The figure shows three views and two pictorial views of one solid part (mm, origin at its lowest corner). Answer the questions. Coordinates: 2 decimals unless noted, no trailing zeros. Order: outer loops, then holes, each group sorted by start corner. A loop starts at its lowest first (then second) coordinate and runs counter-clockwise, first axis right, second up. Notation, with made-up numbers: (11, 40) - (58, 40) arc R28 ccw to (58, 64) - close; hole circle Ø2 at (73.5, -12.5). An arc over 180 degrees is marked (long way). Use one line per item in the form item = value. Start each with the question number.
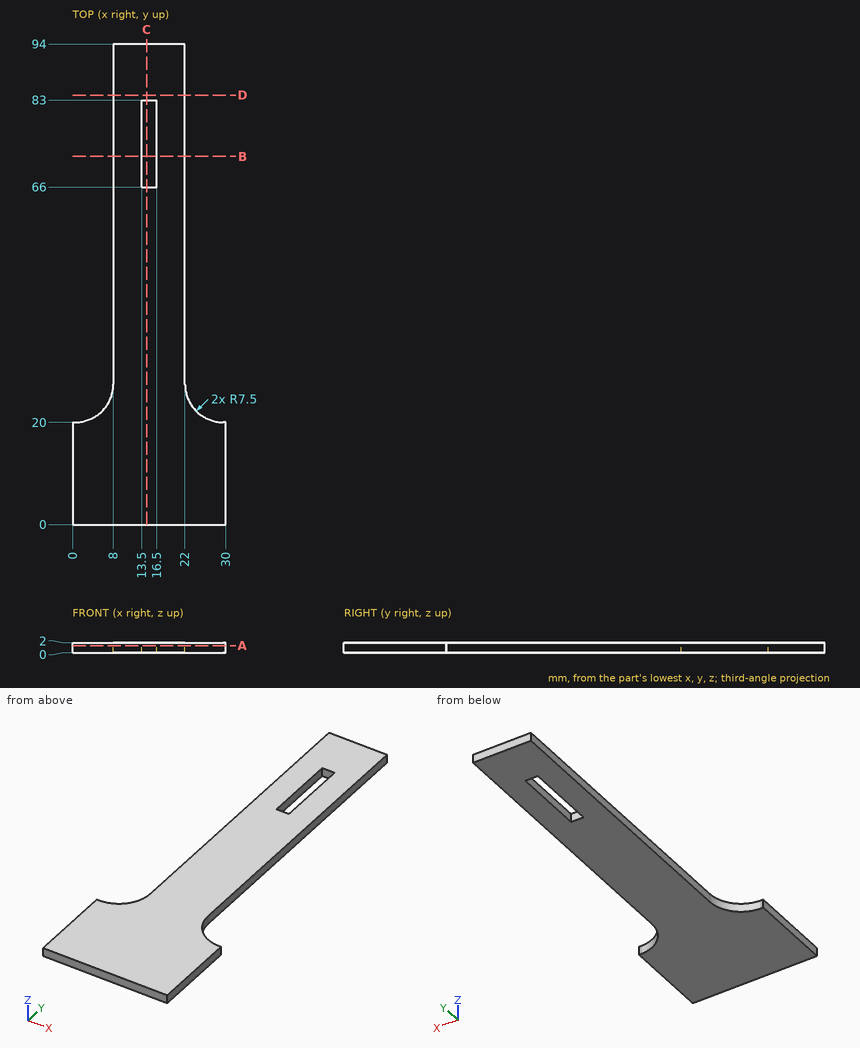
Q1. Given P1, Ø0.6, axis at y = 75.5, z = 0.5, coming from the -X side; P2, Ø0.6, axis at x = 14.5, z = 1, coming from the -Y side; P3, Ø1, axis at y = 72.5, z = 1.5, coming from the +X side, each flat-ended and moving along its own axis, determine where each tip first touches the part or whether it passes through.
Q2. A cutting plane is placed at B-B (y = 72). Give the vertices of the cut face in (x, z), then the cut area to 3 significant figures.
Q3. A cutting plane is placed at D-D (y = 84). Give the vertices of the cut face in (x, z), then the cut area to 3 significant figures.
Q4. A cutting plane is placed at C-C (x = 14.5). Give the vertices of the cut face in (y, z).
Q5. Consider probe 1 along X at (y, z) = (78, 0.15); probe 2 along Y at (x, z) = (16, 0.85); probe 3 along X at (y, z) = (43, 1.85). Determine where each line is inside the solid, lowest interval first.
Q6. A cutting plane is placed at A-A (z = 1.4). Give the vertices of the cut face in (x, y).
Result sheet:
q1.P1 = 8
q1.P2 = 0
q1.P3 = 22
q2.outline = (8, 0) - (13.5, 0) - (13.5, 2) - (8, 2) - close; (16.5, 0) - (22, 0) - (22, 2) - (16.5, 2) - close
q2.area = 22.0 mm^2
q3.outline = (8, 0) - (22, 0) - (22, 2) - (8, 2) - close
q3.area = 28.0 mm^2
q4.outline = (0, 0) - (66, 0) - (66, 2) - (0, 2) - close; (83, 0) - (94, 0) - (94, 2) - (83, 2) - close
q5.probe_1 = 8 to 13.5, 16.5 to 22
q5.probe_2 = 0 to 66, 83 to 94
q5.probe_3 = 8 to 22
q6.outline = (0, 0) - (30, 0) - (30, 20) - (29.5, 20) arc R7.5 cw to (22, 27.5) - (22, 94) - (8, 94) - (8, 27.5) arc R7.5 cw to (0.5, 20) - (0, 20) - close; hole (13.5, 66) - (16.5, 66) - (16.5, 83) - (13.5, 83) - close
